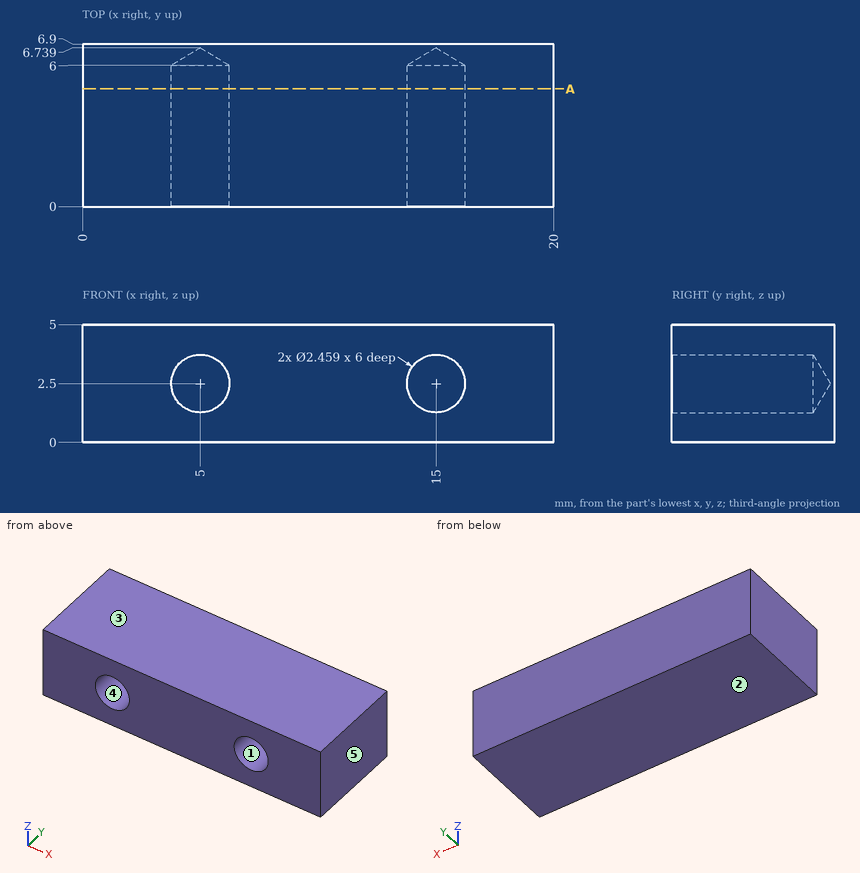
Drawing for the job (mm, zero at the part's lowest x, y, z). A direction names the side the tool comes from. Give positions to 0.01 mm unless a question says otherwise; leave off trailing zeros. Order: outer loops, then holes, each group sorted by start corner. A loop starts at its lowest first (then second) coordinate and runs counter-clockwise, first axis right, second up. Notation, with made-up numbers: M 11,-5.75 L 32,-5.75 A20 cw 32,19.25 Z; hole C 60,-24 d5. An arc over 180 degrees is marked long. Write item = value, one per line. Start each with the question number.
(1) Probe L1, parallel to X at y = 3.4, z = 2.5; L2, parallel to Z at x = 15, y = 4.05; L3, parallel to X at y = 3, z = 3.55. List the from-to ranges inside material, lowest first. Write a range as [from, to].
(2) Slice it at A-A on y = 5. Write the cut outline in (x, z).
(3) Pin check, flat tip, straight feed: pin 1 Ø1.5 at (x, z) = (5, 2.5) entering from -Y. Stop position of the tip, or through.
(4) Which spindle directions (+Z, -Z, +X, -X, +Y, -Y) get a long thin tool onto all of the face, cutting with end or side? Do the marked faces 4 and 5. Say none if no direction does.
(5) Two-plate mould, pull along Z, no slides. Class the marked faces 1, 2 and 3: released by +Z, released by -Z, zero draft, split by the parting line, or undercut.
Responses:
q1.L1 = [0, 3.77], [6.23, 13.77], [16.23, 20]
q1.L2 = [0, 1.27], [3.73, 5]
q1.L3 = [0, 4.36], [5.64, 14.36], [15.64, 20]
q2.outline = M 0,0 L 20,0 L 20,5 L 0,5 Z; hole C 5,2.5 d2.46; hole C 15,2.5 d2.46
q3.pin_1 = 6.29
q4.face_4 = -Y
q4.face_5 = +Z, -Z, +X, +Y, -Y
q5.face_1 = undercut
q5.face_2 = released by -Z
q5.face_3 = released by +Z
